Source: CAD feature listing. Evaluate the final solid. Frame: model axes, mm. Give positions to 0.01 mm unless a question says otherwise; leave off trailing zeros. Write each loop counter-clockwise with the first axis right and the second up, starting at its lowest first coordinate (ties: lowest second). Pieces come first, ordered by that corner, then holes.
Autodesk Inventor part; units mm, degrees
ref_plane "Plano de trabajo1" through (0, 0, 5) normal (0, 0, 1) x (1, 0, 0)
ref_plane "YZ Plane" through (0, 0, 0) normal (1, 0, 0) x (0, 1, 0)
ref_plane "XZ Plane" through (0, 0, 0) normal (0, 1, 0) x (-1, 0, 0)
sketch "Boceto1" plane through (0, 0, 0) normal (0, 0, 1) x (1, 0, 0)
  circle A0 centre (0, 0) radius 7.5
  dimension "d0" = 15
extrude "Extrusión1" add sketch "Boceto1" along normal mid plane 84
ref_plane "Plano de trabajo1" through (0, 0, 5) normal (0, 0, 1) x (1, 0, 0)
sketch "Boceto3" plane through (0, 0, 5) normal (0, 0, 1) x (1, 0, 0)
  circle A0 centre (0, 0) radius 7.5
  line L0 (0, 7.5) -> (0, 6)
  line L1 (0, 6) -> (4.5, 6)
  line L2 (0, 6) -> (-4.5, 6)
  dimension "d4" = 1.5
extrude "Extrusión2" cut sketch "Boceto3" along normal blind 10 contours L1 L0 A0 | A0 L0 L2
properties part number "Eje_engrane"
1. Cut plane A-A, the plane x = 3. Return the cut outline in (y, z), then the cut area to 3 significant figures.
2. Cut plane C-C, the plane z = 2.5. Return the cut outline in (x, y), then the cut area to 3 significant figures.
3. Mould query, pull axis Z, two halves, no side actions, for faces 1 (the flat face through (0, 0, -42)), 2 (the flat face through (0, 0, 42)), 3 (the flat face through (0, 7, 5)), 4 (the cylindrical face through (-1.63, -7.32, 0.59)). Classes: +Z half, -Z half, draft (parallel to the pull), parting line (faces both ways), or undercut.
4. Contact query for flat-ended pins moving along their axis: P1, Ø3, axis at x = -5, z = -33, coming from the -Y side; P2, Ø2, axis at y = 6, z = -20.5, coming from the +X side; P3, Ø5, axis at y = 4.5, z = -13.5, coming from the -X side. Output: stop coordinate, or through.
5. Line query: L1, parallel to X at y = 0.25, z = 24; L2, parallel to Y at x = -0.5, z = -20; L3, parallel to X at y = 6, z = -34.5. Output: solid intervals per line, ascending.
6. Cut plane D-D, the plane x = 6.25. Return the cut outline in (y, z), then the cut area to 3 significant figures.
7. Cut plane B-B, the plane y = 4.5. Return the cut outline in (x, z).
Response values:
1. outline: (-6.87, -42) - (6.87, -42) - (6.87, 5) - (6, 5) - (6, 15) - (6.87, 15) - (6.87, 42) - (-6.87, 42) - close
1. area: 1,150 mm2
2. outline: circle Ø15 at (0, 0)
2. area: 177 mm2
3. face 1: -Z half
3. face 2: +Z half
3. face 3: undercut
3. face 4: draft
4. P1: stops at y = -6.63
4. P2: stops at x = 5.59
4. P3: stops at x = -7.23
5. L1: x = -7.5 to 7.5
5. L2: y = -7.48 to 7.48
5. L3: x = -4.5 to 4.5
6. outline: (-4.15, -42) - (4.15, -42) - (4.15, 42) - (-4.15, 42) - close
6. area: 696 mm2
7. outline: (-6, -42) - (6, -42) - (6, 42) - (-6, 42) - close
